Could you check a few things on this model? Use its own coordinates, in mm. Face numbers are marked on the shaded views. A direction names the side the tool comes from. Coordinates: 2 decimals unless noted, no trailing zeros. Write each loop counter-clockwise with the first axis right and the second up, starting at its lowest first coordinate (ties: lowest second). Pieces come first, ordered by that corner, then holes. Notation, with made-up numbers: (0, 6) - (38, 6) arc R18 cw to (38, 30) - close; hole circle Ø5 at (56.5, -37.75). An arc over 180 degrees is marked (long way). Answer as a JSON object with one key per item and string values. Group by question number.
1) If we section it at A-A (x = 5): Write out the boundary of the cut face in (y, z), plus the area to 3 significant figures.
2) On a 3-axis mill with a long thin cutter (end or side, diameter ignored), from which of +Z, -Z, +X, -X, +Y, -Y can I reach the whole of each face in a straight line? I mean the marked faces 1, 2, 3 and 4. Say none if no direction works.
3) Will these pins go through, and if not, where does the flat tip stop? pin 1 Ø0.7 at (y, z) = (-1.5, -0.5) entering from +X; pin 2 Ø1.5 at (x, y) = (13.5, 1) entering from +Z; pin 3 Ø1.5 at (x, z) = (31, 1.5) entering from +Y.
4) If we section it at B-B (x = 22.5): Write out the boundary of the cut face in (y, z), plus the area to 3 significant figures.
5) Please list where these lines run through material, in increasing order: line 1 along Y through (x, z) = (7.5, 0.15); line 2 along X through (y, z) = (-0.3, 1.8); line 3 along Y through (x, z) = (22.5, 0.4).
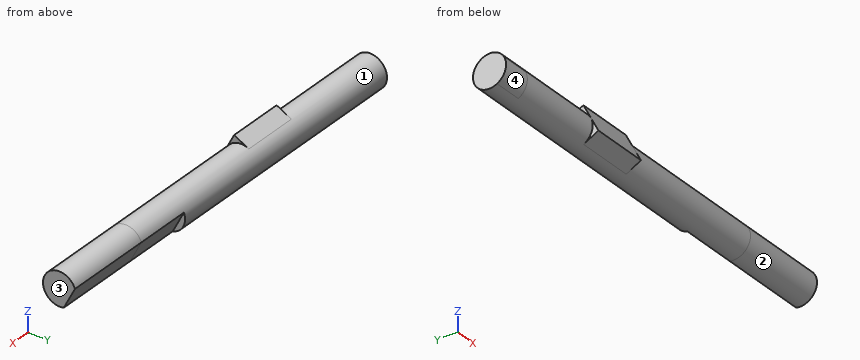
Autodesk Inventor part; units mm, degrees
ref_plane "YZ Plane" through (0, 0, 0) normal (1, 0, 0) x (0, 1, 0)
ref_plane "XZ Plane" through (0, 0, 0) normal (0, 1, 0) x (-1, 0, 0)
ref_plane "XY Plane" through (0, 0, 0) normal (0, 0, 1) x (1, 0, 0)
sketch "Sketch1" plane through (0, 0, 0) normal (1, 0, 0) x (0, 1, 0)
  circle A0 centre (0, 0) radius 1.4986
  dimension "d0" = 2.9972
extrude "Extrusion1" add sketch "Sketch1" along normal blind 25.4
ref_plane "Work Plane1" through (7.81, -18.8269, 9.6237) normal (1, 0, 0) x (0, 0.4551504, 0.8904146)
sketch "Sketch2" plane through (7.81, -18.8269, 9.6237) normal (1, 0, 0) x (0, 0.4551504, 0.8904146)
  line L0 (0, -21.144) -> (-1.4986, -21.144) construction
  circle A0 centre (0, -21.144) radius 1.4986 construction
  line L1 (-1.4986, -21.144) -> (-1.4986, -19.6454)
  line L2 (-1.4986, -19.6454) -> (1.4986, -19.6454)
  line L3 (1.4986, -19.6454) -> (1.4986, -21.144)
  line L4 (-1.4986, -21.144) -> (1.4986, -21.144)
extrude "Extrusion2" add sketch "Sketch2" along normal blind 5.08
sketch "Sketch3" plane through (25.4, 0, 0) normal (1, 0, 0) x (0, 0, -1)
  circle A0 centre (0, 0) radius 1.4986
extrude "Extrusion3" add sketch "Sketch3" along normal blind 1.27
sketch "Sketch4" plane through (26.67, 0, 0) normal (1, 0, 0) x (0, 0, -1)
  line L0 (-0.5404, 1.3993) -> (1.4507, 0.3815)
  arc A0 (-10.1641, -17.4276) -> (-8.173, -18.4454) centre (-9.6237, -18.8269) ccw
  line L1 (-10.1641, -17.4276) -> (-8.173, -18.4454)
  line L2 (-2.0165, -0.6523) -> (-0.6821, -1.3344)
  arc A1 (1.4507, 0.3815) -> (-0.5404, 1.3993) centre (0, 0) ccw
extrude "Extrusion4" cut sketch "Sketch4" against normal blind 5.08 contours A1 L0
sketch "Sketch5" plane through (26.67, 0, 0) normal (1, 0, 0) x (0, 0, -1)
  line L0 (1.449, 0.3824) -> (-0.5387, 1.3984)
  line L1 (1.449, 0.3824) -> (-0.5387, 1.3984)
  arc A0 (-0.5387, 1.3984) -> (1.449, 0.3824) centre (0, 0) ccw
extrude "Extrusion5" add sketch "Sketch5" along normal blind 7.9375
sketch "Sketch6" plane through (0, 0, 0) normal (-1, 0, 0) x (0, 0, 1)
  arc A0 (-1.3344, -0.6821) -> (0.6821, -1.3344) centre (0, 0) ccw
  circle A1 centre (0, 0) radius 1.4986
extrude "Extrusion6" add sketch "Sketch6" along normal blind 2.54
properties part number "Shaft" material "PAEK Plastic"
Here are the results:
{
 "1": {"outline": "circle Ø3 at (0, 0)", "area": "7.06 mm²"},
 "2": {"face 1": "none", "face 2": "+X", "face 3": "+Z, -Z, +X, +Y, -Y", "face 4": "-X, -Y"},
 "3": {"pin 1": "stops at x = 34.61", "pin 2": "stops at z = 1.48", "pin 3": "stops at y = 1.3"},
 "4": {"outline": "(0.38, -1.45) - (1.4, 0.54) arc R1.5 ccw (long way) to start", "area": "6.28 mm²"},
 "5": {"line 1": "y = -1.49 to 1.49", "line 2": "x = 7.81 to 12.89", "line 3": "y = -1.44 to 1.33"}
}
